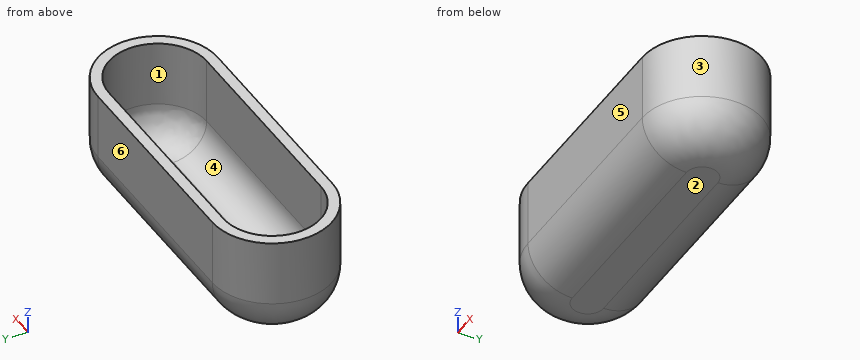
from build123d import *

# Parameters (mm, degrees)
F1_DEPTH = 25
F2_DEPTH = 25
F3_R     = 10
F4_T     = -2.5


with BuildPart() as f1:
    # F0 (on Top) → F1 (new body)
    with BuildSketch(Plane.XY):
        with BuildLine():
            Line((-47.356255, -13.546846), (0, -13.546846))
            ThreePointArc((0, -13.546846), (13.546846, 0), (0, 13.546846))
            Line((0, 13.546846), (-47.356255, 13.546846))
            ThreePointArc((-47.356255, 13.546846), (-60.903101, 0), (-47.356255, -13.546846))
        make_face()
    extrude(amount=F1_DEPTH)

    # F0 (on Top) → F2 (join)
    with BuildSketch(Plane.XY):
        with BuildLine():
            Line((-47.356255, -13.546846), (0, -13.546846))
            ThreePointArc((0, -13.546846), (13.546846, 0), (0, 13.546846))
            Line((0, 13.546846), (-47.356255, 13.546846))
            ThreePointArc((-47.356255, 13.546846), (-60.903101, 0), (-47.356255, -13.546846))
        make_face()
    extrude(amount=F2_DEPTH)

    # F3
    f3_edges = [f1.edges().sort_by_distance(p)[0] for p in [
        (-60.903101, 0, 0),
    ]]
    fillet(f3_edges, radius=F3_R)

    # F4
    f4_openings = [f1.faces().sort_by_distance(p)[0] for p in [
        (-23.678128, 0, 25),
    ]]
    offset(amount=F4_T, openings=f4_openings)


solid = f1.part
Here's how the part is built. I have some questions about the finished solid (model axes, mm). Face numbers are marked on the shaded views. A direction names the side the tool comes from. Round coordinates to 2 decimals unless told otherwise and drop trailing zeros. Loops run counter-clockwise (first coordinate to the right, second up) from the corner with the lowest first, then second, coordinate; pieces in that order, holes last.
1. If we section it at B-B on x = -44.5: Write out the boundary of the cut face in (y, z), plus the area to 3 significant figures.
Answer list:
outline: (-13.55, 10) arc R10 ccw to (-3.55, 0) - (3.55, 0) arc R10 ccw to (13.55, 10) - (13.55, 25) - (11.05, 25) - (11.05, 10) arc R7.5 cw to (3.55, 2.5) - (-3.55, 2.5) arc R7.5 cw to (-11.05, 10) - (-11.05, 25) - (-13.55, 25) - close
area: 161 mm2
2. For P1, Ø5.5, axis at x = -35, y = 1.5, coming from the +Z side; P2, Ø10, axis at y = 10, z = 19.5, coming from the +X side; P3, Ø5, axis at y = 8, z = 15, coming from the -X side; P4, Ø6, axis at y = 1.5, z = 18, coming from the +X side, each with a flat end and sliding along its axis, tell me the tip position at first contact or that it passes through.
Answer list:
P1: stops at z = 2.53
P2: stops at x = 12.59
P3: stops at x = -59.74
P4: stops at x = 13.55
3. If we section it at A-A on z = 19: Write out the boundary of the cut face in (x, y).
Answer list:
outline: (-47.36, -13.55) - (0, -13.55) arc R13.55 ccw to (0, 13.55) - (-47.36, 13.55) arc R13.55 ccw to start; hole (-47.36, -11.05) - (0, -11.05) arc R11.05 ccw to (0, 11.05) - (-47.36, 11.05) arc R11.05 ccw to start
4. If I drill on line 1 along Y through (x, z) = (-47.5, 10.5); line 2 along Z through (x, y) = (-10, 2.5); line 3 along X through (y, z) = (3.5, 6), over which ranges is the centre line in solid material (lowest first)?
Answer list:
line 1: y = -13.55 to -11.05, 11.05 to 13.55
line 2: z = 0 to 2.5
line 3: x = -59.58 to -56.61, 9.25 to 12.22
5. Which directions (+Z, -Z, +X, -X, +Y, -Y) give clear straight access to the entire face, cutting with the end or side of a thin tool? Please do the marked faces 1 and 2.
Answer list:
face 1: +Z
face 2: -Z, +X, -X, +Y, -Y
6. We'd pull the mould along Y, two halves only. Please class the marked faces 3, 4, 5 and 6: +Y half, -Y half, draft (parallel to the pull), parting line (faces both ways), or undercut.
Answer list:
face 3: parting line
face 4: undercut
face 5: -Y half
face 6: +Y half
